The model under review builds one solid part; all positions refer to its coordinate system, in mm. A direction names the side the tool comes from. Give positions to 0.01 mm unless a question says otherwise; leave off trailing zeros. Write each loop counter-clockwise with the first axis right and the second up, starting at its lowest first coordinate (ties: lowest second). Pieces come first, ordered by that corner, then holes. Notation, with made-up numbers: (10, -30) - (69, -30) arc R14 cw to (69, -25) - close; hole circle Ø11 at (34.5, 83.25). An arc over 180 degrees is marked (long way). Write item = value, one per line.
Solid Edge part; units mm, degrees
sketch "Sketch1" plane through (0, 0, 0) normal (1, 0, 0) x (0, 1, 0)
  line L0 (0, -2.1082) -> (0, 2.1082)
  arc A0 (0, 2.1082) -> (6.9469, -2.1082) centre (-0.3606, -6.3169) cw
  line L1 (0, -2.1082) -> (6.9469, -2.1082)
revolve "RevolvedProtrusion1" add sketch "Sketch1" angle 360 about axis through (0, 0, -14.7796) along (0, 0, 1)
sketch "Sketch2" plane through (0, 0, -2.1082) normal (0, 0, -1) x (0, 1, 0)
  circle A0 centre (0, 0) radius 3.175
extrude "Protrusion1" add sketch "Sketch2" along normal blind 25.4
sketch "Sketch3" plane through (-0.6032, 0.3606, 4.2164) normal (0, 0, 1) x (1, 0, 0)
  line L0 (-0.7716, 2.0206) -> (1.978, 2.0206)
  line L1 (3.3529, -0.3606) -> (1.978, 2.0206)
  line L2 (1.978, -2.7419) -> (3.3529, -0.3606)
  line L3 (-0.7716, -2.7419) -> (1.978, -2.7419)
  line L4 (-2.1464, -0.3606) -> (-0.7716, -2.7419)
  line L5 (-0.7716, 2.0206) -> (-2.1464, -0.3606)
extrude "ExtrudedCutout_11" cut sketch "Sketch3" against normal blind 6.3246
cosmetic_thread "Thread_1" thread depth 23.8252
properties part number "218623"
1. For line 1 (Y direction, x = -2.25, z = -1.5); line 2 (Z direction, x = 2.5, y = 0); line 3 (Z direction, x = -5.75, y = -1), list the stretches that pass through material, from the lowest coordinate up. Write a range as from..to.
Findings below:
line_1 = -6.16..-0.87, 0.87..6.16
line_2 = -27.51..-2.11
line_3 = -2.11..-0.6
2. Machinability: for faces 1 (the conical face through (2.88, 1.83, -2.11)), 2 (the flat face through (2.072, 1.174, -0.199)), which of the approach directions +Z, -Z, +X, -X, +Y, -Y give a long, thin tool a straight path to every point of the face, cutting with its end or side? Answer none if there is none.
Findings below:
face_1 = -Z
face_2 = +Z
3. Take a section at A-A on z = -15.25. Give the boundary of the cut face in (x, y) (3 decimals), and give its area (3 significant figures).
Findings below:
outline = circle Ø6.35 at (0, 0)
area = 31.7 mm²
4. Draft analysis for pull direction X (two halves, no side actions). For faces 3 (the flat face through (2.05, -1.21, -0.2)), 4 (the flat face through (0, 0, -27.508)), 5 (the cylindrical face through (3.1, -0.69, -14.63)), state which applies: +X half, -X half, draft (parallel to the pull), parting line (faces both ways), or undercut.
Findings below:
face_3 = undercut
face_4 = draft
face_5 = parting line
5. Insertion check: P1, Ø4, axis at x = 0, y = -1, coming from the +Z side; P2, Ø0.8, axis at x = 0, z = 0, coming from the +Y side; P3, Ø6, axis at x = 2, z = -9, coming from the -Y side (3 decimals); P4, Ø2, axis at y = 0.5, z = -7.5, coming from the -X side (3 decimals). Each pin has a flat end and moves straight along its axis. Give the tip position at first contact, or say it passes through.
Findings below:
P1 = 1.66
P2 = 5.65
P3 = -3.175
P4 = -3.175
